Part model, mm, in its own coordinate system. Give positions to 0.01 mm unless a question says otherwise; leave off trailing zeros. Write each loop counter-clockwise with the first axis right and the second up, starting at its lowest first coordinate (ties: lowest second). Pieces come first, ordered by that corner, then holes. Notation, with made-up numbers: M -38,45 L 2,45 A20 cw 2,82 Z; hole C -4.75,14.5 d4. An arc over 180 degrees is marked long. Write item = value, one per line. Start each with the question number.
from build123d import *

# Parameters (mm, degrees)
SKETCH_1_W          = 22
SKETCH_1_H          = 42
SKETCH_1_W_2        = 2
SKETCH_1_H_2        = 38
EXTRUDE_1_DEPTH     = 3
SKETCH_2_R          = 1.5
CUT_EXTRUDE_1_DEPTH = 10


with BuildPart() as part:
    # 草图1 → 凸台-拉伸1 (new body)
    with BuildSketch(Plane.XY):
        Rectangle(SKETCH_1_W, SKETCH_1_H)
        with Locations((-12, 0)):
            Rectangle(SKETCH_1_W_2, SKETCH_1_H_2)
        with Locations((12, 0)):
            Rectangle(SKETCH_1_W_2, SKETCH_1_H_2)
    extrude(amount=EXTRUDE_1_DEPTH)

    # 草图2 → 切除-拉伸1 (cut)
    with BuildSketch(Plane.XY.offset(3)):
        with Locations((5.3, -7.6)):
            Circle(SKETCH_2_R)
        with Locations((5.3, 7.6)):
            Circle(SKETCH_2_R)
        with BuildLine():
            Line((-7.45, -10), (-7.45, 10))
            ThreePointArc((-7.45, 10), (-6.45, 11), (-5.45, 10))
            Line((-5.45, 10), (-5.45, -10))
            ThreePointArc((-5.45, -10), (-6.45, -11), (-7.45, -10))
        make_face()
    extrude(amount=-CUT_EXTRUDE_1_DEPTH, mode=Mode.SUBTRACT)


solid = part.part
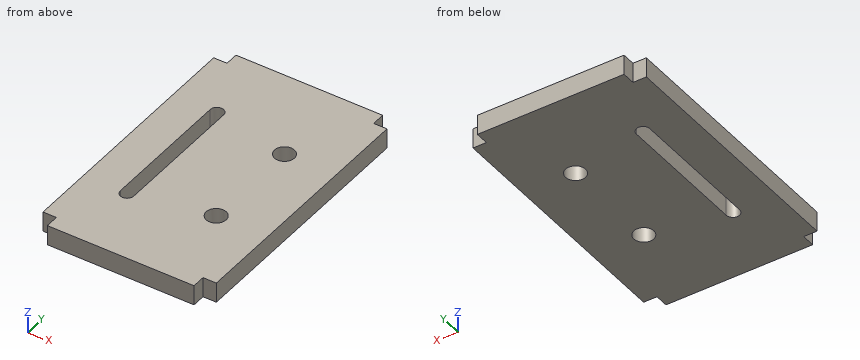
Q1. Slice it at C-C (x = 5.3). Give the cut face in (y, z).
Q2. Drop flat-ended pins along their axis: P1, Ø1.6, axis at x = 12.5, z = 1.5, coming from the +Y side; P2, Ø1, axis at y = -20, z = 2, coming from the +X side; P3, Ø1, axis at y = -20, z = 2, coming from the -X side. Give the stop position or say it passes through.
Q3. Slice it at D-D (y = -1). Give the cut face in (x, z).
Q4. Probe line 1 along Y through (x, z) = (5.3, 1.8); line 2 along X through (y, z) = (-5.5, 2.3); line 3 along Y through (x, z) = (4, 1.55). List the from-to ranges inside material, lowest first.
Q5. Slice it at A-A (y = 7.6). Give the cut face in (x, z).
Q6. Slice it at B-B (z = 2.6). Give the cut face in (x, y).
Working result:
q1.outline = M -21,0 L -9.1,0 L -9.1,3 L -21,3 Z; M -6.1,0 L 6.1,0 L 6.1,3 L -6.1,3 Z; M 9.1,0 L 21,0 L 21,3 L 9.1,3 Z
q2.P1 = 19
q2.P2 = 11
q2.P3 = -11
q3.outline = M -13,0 L -7.45,0 L -7.45,3 L -13,3 Z; M -5.45,0 L 13,0 L 13,3 L -5.45,3 Z
q4.line_1 = -21 to -9.1, -6.1 to 6.1, 9.1 to 21
q4.line_2 = -13 to -7.45, -5.45 to 13
q4.line_3 = -21 to -8.35, -6.85 to 6.85, 8.35 to 21
q5.outline = M -13,0 L -7.45,0 L -7.45,3 L -13,3 Z; M -5.45,0 L 3.8,0 L 3.8,3 L -5.45,3 Z; M 6.8,0 L 13,0 L 13,3 L 6.8,3 Z
q6.outline = M -13,-19 L -11,-19 L -11,-21 L 11,-21 L 11,-19 L 13,-19 L 13,19 L 11,19 L 11,21 L -11,21 L -11,19 L -13,19 Z; hole M -7.45,-10 A1 ccw -5.45,-10 L -5.45,10 A1 ccw -7.45,10 Z; hole C 5.3,-7.6 d3; hole C 5.3,7.6 d3
